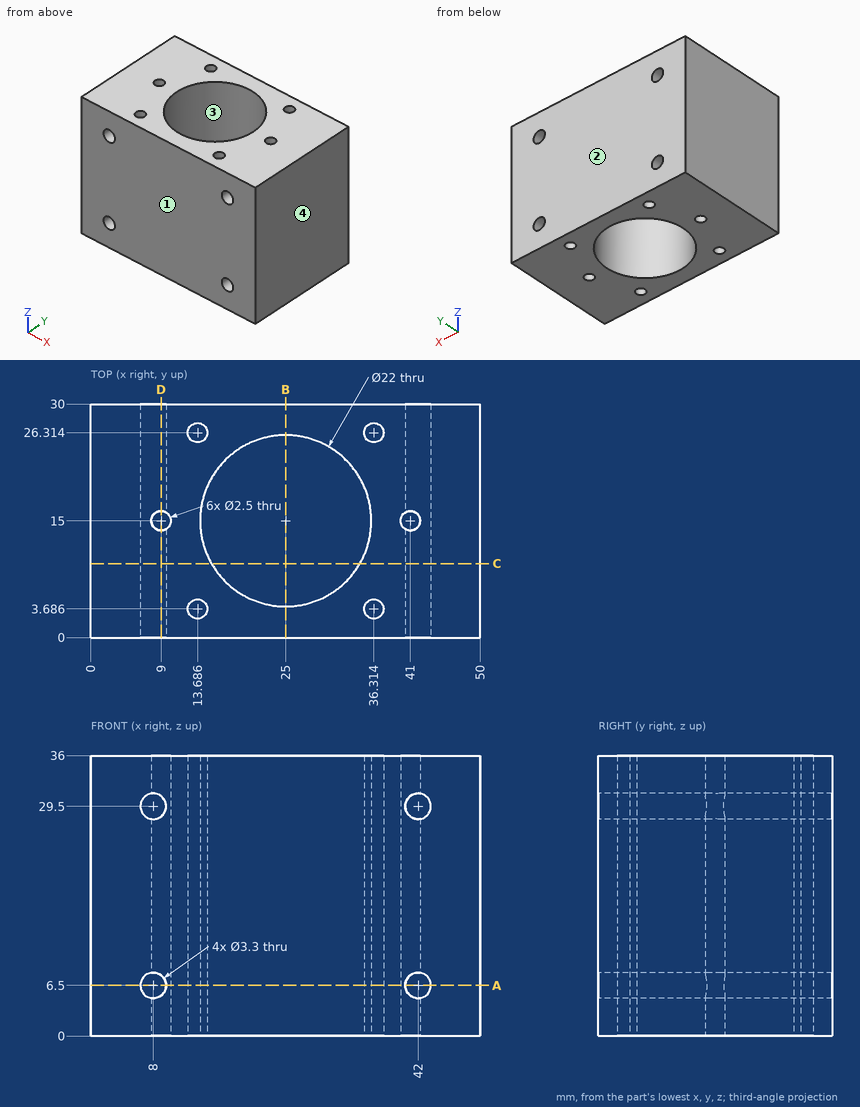
Here's the drawing with two shaded views (mm, measured from the low corner). I have some questions. Coordinates: 2 decimals unless noted, no trailing zeros. Order: outer loops, then holes, each group sorted by start corner. A loop starts at its lowest first (then second) coordinate and runs counter-clockwise, first axis right, second up. Notation, with made-up numbers: (37, 88) -> (42, 88) arc R30 ccw to (42, 127) -> close; hole circle Ø8 at (29, 59.5). An arc over 180 degrees is marked (long way). One line per question, with ' | ' between items.
Q1. Thinking about a two-plate mould opening in Y: for the marked faces 1, 2, 3 and 4, which applies, pulls with the +Y half, pulls with the -Y half, needs draft (parallel to the pull), parting line crosses it, or undercut?
Return value:
face 1: pulls with the -Y half | face 2: pulls with the +Y half | face 3: undercut | face 4: needs draft
Q2. Imagine slicing it at C-C on y = 9.5. Please give me the cut outline in (x, z).
Return value:
outline: (0, 0) -> (15.47, 0) -> (15.47, 36) -> (0, 36) -> close; (34.53, 0) -> (50, 0) -> (50, 36) -> (34.53, 36) -> close; hole circle Ø3.3 at (8, 6.5); hole circle Ø3.3 at (8, 29.5); hole circle Ø3.3 at (42, 6.5); hole circle Ø3.3 at (42, 29.5)
Q3. Imagine slicing it at A-A on z = 6.5. Please give me the cut outline in (x, y).
Return value:
outline: (0, 0) -> (6.35, 0) -> (6.35, 30) -> (0, 30) -> close; (9.65, 0) -> (40.35, 0) -> (40.35, 13.93) arc R1.25 cw to (40.35, 16.07) -> (40.35, 30) -> (9.65, 30) -> (9.65, 16.07) arc R1.25 cw to (9.65, 13.93) -> close; (43.65, 0) -> (50, 0) -> (50, 30) -> (43.65, 30) -> close; hole circle Ø2.5 at (13.69, 3.69); hole circle Ø2.5 at (13.69, 26.31); hole circle Ø22 at (25, 15); hole circle Ø2.5 at (36.31, 3.69); hole circle Ø2.5 at (36.31, 26.31)
Q4. If I drill on L1, parallel to Y at x = 25.5, z = 5; L2, parallel to Z at x = 8, y = 7; L3, parallel to Y at x = 41, z = 21, over which ranges is the centre line in solid material (lowest first)?
Return value:
L1: 0 to 4.01, 25.99 to 30 | L2: 0 to 4.85, 8.15 to 27.85, 31.15 to 36 | L3: 0 to 13.75, 16.25 to 30
Q5. Imagine slicing it at B-B on x = 25. Please give me the cut outline in (y, z), and give its area (3 significant figures).
Return value:
outline: (0, 0) -> (4, 0) -> (4, 36) -> (0, 36) -> close; (26, 0) -> (30, 0) -> (30, 36) -> (26, 36) -> close | area: 288 mm²
Q6. Imagine slicing it at D-D on x = 9. Please give me the cut outline in (y, z).
Return value:
outline: (0, 0) -> (13.75, 0) -> (13.75, 5.19) -> (0, 5.19) -> close; (0, 7.81) -> (13.75, 7.81) -> (13.75, 28.19) -> (0, 28.19) -> close; (0, 30.81) -> (13.75, 30.81) -> (13.75, 36) -> (0, 36) -> close; (16.25, 0) -> (30, 0) -> (30, 5.19) -> (16.25, 5.19) -> close; (16.25, 7.81) -> (30, 7.81) -> (30, 28.19) -> (16.25, 28.19) -> close; (16.25, 30.81) -> (30, 30.81) -> (30, 36) -> (16.25, 36) -> close
